from build123d import *

# Parameters (mm, degrees)
SKETCH_W     = 29
SKETCH_H     = 20
SKETCH_R     = 1
PAD_DEPTH    = 1
FILLET_R     = 1.25
SKETCH001_W  = 5
SKETCH001_H  = 15
PAD001_DEPTH = 5


with BuildPart() as part:
    # Sketch → Pad (new body)
    with BuildSketch(Plane.XY):
        Rectangle(SKETCH_W, SKETCH_H)
        with Locations((-12.48, -8.095)):
            Circle(SKETCH_R, mode=Mode.SUBTRACT)
        with Locations((-12.48, 8.095)):
            Circle(SKETCH_R, mode=Mode.SUBTRACT)
    extrude(amount=PAD_DEPTH)

    # Fillet
    fillet_edges = [part.edges().sort_by_distance(p)[0] for p in [
        (14.5, -10, 0.5),
        (14.5, 10, 0.5),
        (-14.5, -10, 0.5),
        (-14.5, 10, 0.5),
    ]]
    fillet(fillet_edges, radius=FILLET_R)

    # Sketch001 (on Face5 of Fillet) → Pad001 (join)
    with BuildSketch(Plane.XY.offset(1)):
        with Locations((12, 0)):
            Rectangle(SKETCH001_W, SKETCH001_H)
    extrude(amount=PAD001_DEPTH)


solid = part.part
Here's how the part is built. I have some questions about the finished solid (model axes, mm). A direction names the side the tool comes from. Round coordinates to 2 decimals unless told otherwise and drop trailing zeros. Order: outer loops, then holes, each group sorted by start corner. A loop starts at its lowest first (then second) coordinate and runs counter-clockwise, first axis right, second up. Notation, with made-up numbers: M -22,-25.5 L 22,-25.5 A31 ccw 22,-1.5 Z; hole C 28,23.25 d9. An arc over 180 degrees is marked long. Return JSON: item names as keys, results as strings. Group by question number.
1. On a 3-axis mill with a long thin cutter (end or side, diameter ignored), from which of +Z, -Z, +X, -X, +Y, -Y can I reach the whole of each face in a straight line? I mean faces 1 (the face through (12, -7.5, 3)), 2 (the face through (-14.5, -0.1, 0.5)), 3 (the face through (12, 7.5, 3)), 4 (the face through (9.5, 0, 3)). Say none if no direction works.
2. If we section it at D-D on z = 5.55: List the corners of the cut face in (x, y) for me, then the cut area to 3 significant figures.
3. Please list where these lines run through material, in increasing order: probe 1 along Y at (x, z) = (-12.48, 0.2) (3 decimals); probe 2 along X at (y, z) = (1.5, 5.7); probe 3 along Z at (x, y) = (-5, -8).
4. If we section it at A-A on x = -12.48: List the corners of the cut face in (y, z) for me (3 decimals).
5. If we section it at B-B on y = 4.75: List the corners of the cut face in (x, z) for me.
6. I'm going to push flat-ended pins straight in: pin 1 Ø2 at (y, z) = (0, 2.5) entering from -X; pin 2 Ø10 at (x, y) = (3.5, 3.5) entering from -Z; pin 3 Ø2.5 at (x, y) = (-12.48, -8.095) entering from +Z. Where does each tip first touch, or does it pass through?
7. If we mould it in two halves opening along Y, with no side actions, what happens to faces 5 (the face through (-14.144, 9.624, 0.507)), 6 (the face through (-13.48, 8.14, 0.49)), 7 (the face through (-13.48, -8.05, 0.49)), 8 (the face through (0, 0, 0))? For each: pulls with the +Y half, pulls with the -Y half, needs draft (parallel to the pull), parting line crosses it, or undercut.
8. If we section it at C-C on x = 12: List the corners of the cut face in (y, z) for me.
Reply:
{
 "1": {"face 1": "+Z, +X, -X, -Y", "face 2": "+Z, -Z, -X, +Y, -Y", "face 3": "+Z, +X, -X, +Y", "face 4": "+Z, -X, +Y, -Y"},
 "2": {"outline": "M 9.5,-7.5 L 14.5,-7.5 L 14.5,7.5 L 9.5,7.5 Z", "area": "75.0 mm^2"},
 "3": {"probe 1": "-10 to -9.095, -7.095 to 7.095, 9.095 to 10", "probe 2": "9.5 to 14.5", "probe 3": "0 to 1"},
 "4": {"outline": "M -10,0 L -9.095,0 L -9.095,1 L -10,1 Z; M -7.095,0 L 7.095,0 L 7.095,1 L -7.095,1 Z; M 9.095,0 L 10,0 L 10,1 L 9.095,1 Z"},
 "5": {"outline": "M -14.5,0 L 14.5,0 L 14.5,6 L 9.5,6 L 9.5,1 L -14.5,1 Z"},
 "6": {"pin 1": "x = 9.5", "pin 2": "z = 0", "pin 3": "z = 1"},
 "7": {"face 5": "pulls with the +Y half", "face 6": "undercut", "face 7": "undercut", "face 8": "needs draft"},
 "8": {"outline": "M -10,0 L 10,0 L 10,1 L 7.5,1 L 7.5,6 L -7.5,6 L -7.5,1 L -10,1 Z"}
}
